Autodesk Inventor part; units mm, degrees
ref_plane "YZ Plane" through (0, 0, 0) normal (1, 0, 0) x (0, 1, 0)
ref_plane "XZ Plane" through (0, 0, 0) normal (0, 1, 0) x (-1, 0, 0)
ref_plane "XY Plane" through (0, 0, 0) normal (0, 0, 1) x (1, 0, 0)
sketch "Boceto1" plane through (0, 0, 0) normal (0, 0, 1) x (1, 0, 0)
  line L0 (-200, 150) -> (200, 150)
  line L1 (200, 150) -> (200, -150)
  line L2 (200, -150) -> (-200, -150)
  line L3 (-200, -150) -> (-200, 150)
  point P0 (0, 0)
  point P1 (0, 150)
  point P2 (-200, 0)
  dimension "d0" = 400
  dimension "d1" = 300
extrude "Extrusión1" add sketch "Boceto1" along normal blind 160
sketch "Boceto2" plane through (-200, 150, 0) normal (0, 1, 0) x (1, 0, 0)
  line L0 (400, 0) -> (0, 0) construction
  line L1 (0, 0) -> (0, -160) construction
  line L2 (400, -160) -> (0, -160) construction
  line L3 (400, 0) -> (400, -160) construction
  line L4 (10, -150) -> (10, -10)
  line L5 (10, -10) -> (390, -10)
  line L6 (390, -10) -> (390, -150)
  line L7 (390, -150) -> (10, -150)
  point P0 (200, 0)
  dimension "d4" = 10
extrude "Extrusión2" cut sketch "Boceto2" against normal blind 290
sketch "Boceto3" plane through (0, 0, 160) normal (0, 0, 1) x (1, 0, 0)
  line L0 (-200, -150) -> (200, -150) construction
  line L1 (200, -150) -> (200, 150) construction
  line L2 (200, 150) -> (-200, 150) construction
  line L3 (-200, 150) -> (-200, -150) construction
  circle A0 centre (-120, -80) radius 40
  point P0 (0, 0)
  dimension "d7" = 80
  dimension "d8" = 80
  dimension "d9" = 70
extrude "Extrusión3" cut sketch "Boceto3" against normal blind 10
sketch "Boceto4" plane through (0, 0, 0) normal (0, 0, -1) x (-1, 0, 0)
  circle A0 centre (-140, 100) radius 40
  line L0 (200, -150) -> (-200, -150) construction
  line L1 (200, 150) -> (200, -150) construction
  line L2 (-200, 150) -> (200, 150) construction
  line L3 (-200, -150) -> (-200, 150) construction
  point P0 (0, 0)
  dimension "d12" = 80
  dimension "d13" = 50
  dimension "d14" = 60
extrude "Extrusión4" cut sketch "Boceto4" against normal blind 10
properties part number "caja de cambios"
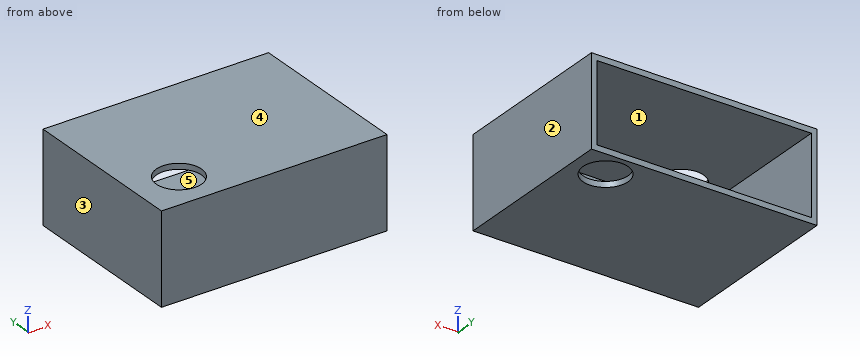
Design review of the part built by this model. Coordinates are the model's own, in mm. Face numbers are marked on the shaded views. A direction names the side the tool comes from. Coordinates: 2 decimals unless noted, no trailing zeros. Order: outer loops, then holes, each group sorted by start corner. A loop starts at its lowest first (then second) coordinate and runs counter-clockwise, first axis right, second up. Notation, with made-up numbers: (79, 30.5) -> (134, 30.5) arc R21 ccw to (134, 63.5) -> close; hole circle Ø7 at (59.5, 13.5). An arc over 180 degrees is marked (long way). Use one line per item in the form item = value. Start each with the question number.
(1) The part is to be moulded in two halves that separate along X. For the marked faces 1, 2 and 3, say which applies: +X half, -X half, draft (parallel to the pull), parting line (faces both ways), or undercut.
(2) Add section C-C on z = 18. State the section outline as (x, y) points, plus the area to 3 significant figures.
(3) For the marked faces 4 and 5, list the 3-axis set-ups (+Z, -Z, +X, -X, +Y, -Y) from which the entire face can be reached by the end or side of a thin tool; tool diameter is ignored.
(4) Add section A-A on x = 172. State the section outline as (y, z) points, plus the area to 3 significant figures.
(5) For probe 1 along X at (y, z) = (-46, 10.5); probe 2 along Y at (x, z) = (140, 3.25); probe 3 along Z at (x, y) = (8, -63.5), list the stretches that pass through material, from the lowest coordinate up.
(6) Insertion check: pin 1 (8 mm diameter, centred on x = -135, y = -90.5, fed in from +Z); pin 2 (3 mm diameter, centred on x = 45, z = 134.5, fed in from +Y); pin 3 (4 mm diameter, centred on x = -34.5, y = 43.5, fed in from -Z). Each pin has a flat end and moves straight along its axis. Give the tip position at first contact, or say it passes through.
(7) Add section D-D on y = -80. State the section outline as (x, z) points.
(8) Add section B-B on y = 36. State the section outline as (x, z) points, plus the area to 3 significant figures.
Answer block:
q1.face_1 = undercut
q1.face_2 = +X half
q1.face_3 = -X half
q2.outline = (-200, -150) -> (200, -150) -> (200, 150) -> (190, 150) -> (190, -140) -> (-190, -140) -> (-190, 150) -> (-200, 150) -> close
q2.area = 9,800 mm²
q3.face_4 = +Z, +X, -X, +Y, -Y
q3.face_5 = +Y
q4.outline = (-150, 0) -> (76, 0) -> (76, 10) -> (-140, 10) -> (-140, 150) -> (150, 150) -> (150, 160) -> (-150, 160) -> close; (124, 0) -> (150, 0) -> (150, 10) -> (124, 10) -> close
q4.area = 6,920 mm²
q5.probe_1 = -200 to -190, 190 to 200
q5.probe_2 = -150 to 60, 140 to 150
q5.probe_3 = 0 to 10, 150 to 160
q6.pin_1 = 10
q6.pin_2 = -140
q6.pin_3 = 0
q7.outline = (-200, 0) -> (200, 0) -> (200, 160) -> (-80, 160) -> (-80, 150) -> (190, 150) -> (190, 10) -> (-190, 10) -> (-190, 150) -> (-160, 150) -> (-160, 160) -> (-200, 160) -> close
q8.outline = (-200, 0) -> (200, 0) -> (200, 160) -> (-200, 160) -> close; hole (-190, 10) -> (190, 10) -> (190, 150) -> (-190, 150) -> close
q8.area = 10,800 mm²
